Geometry: see drawing. Coordinates: mm, zero at the bounding-box minimum. A direction names the side the tool comes from. Coordinates: 2 decimals unless noted, no trailing zeros. Write each loop counter-clockwise with the first axis right and the second up, starting at its lowest first coordinate (ties: lowest second). Pieces come first, ordered by that corner, then holes. Notation, with made-up numbers: M -22,17.25 L 34,17.25 A18 ccw 34,26.25 Z; hole C 76,9.25 d2. An arc over 180 degrees is marked long. One line per item, written item: value. Start each with the question number.
Item 1: Cut plane C-C, the plane y = 45. Output: boundary loops of the cut face in (x, z).
Item 2: Cut plane A-A, the plane z = 20.32. Output: boundary loops of the cut face in (x, y).
Item 3: Set-up query: the marked faces 1 and 2. Return all of +Z, -Z, +X, -X, +Y, -Y with unobstructed straight access to the full face (end or side cutting, diameter ignored); none if empty.
Item 4: Cut plane B-B, the plane x = 0.75. Output: boundary loops of the cut face in (y, z), then the cut area to 3 significant figures.
Item 5: Mould query, pull axis Z, two halves, no side actions, for the marked faces 3, 4, 5 and 6. Classes: released by +Z, released by -Z, zero draft, split by the parting line, or undercut.
Item 6: Cut plane D-D, the plane z = 38.5. Output: boundary loops of the cut face in (x, y).
Item 7: Pin query (flat end, axial travel): P1, Ø1, axis at x = 3, z = 36, coming from the +Y side; P2, Ø1.9, axis at x = 4.5, z = 23, coming from the -Y side. Return the tip coordinate at first contact, or that it passes through.
Item 8: Ray query, L1, parallel to Y at x = 4, z = 20.32; L2, parallel to Z at x = 5.75, y = 3; L3, parallel to Y at x = 4, z = 18. Return the intervals inside material, ascending. Write a range as from..to.
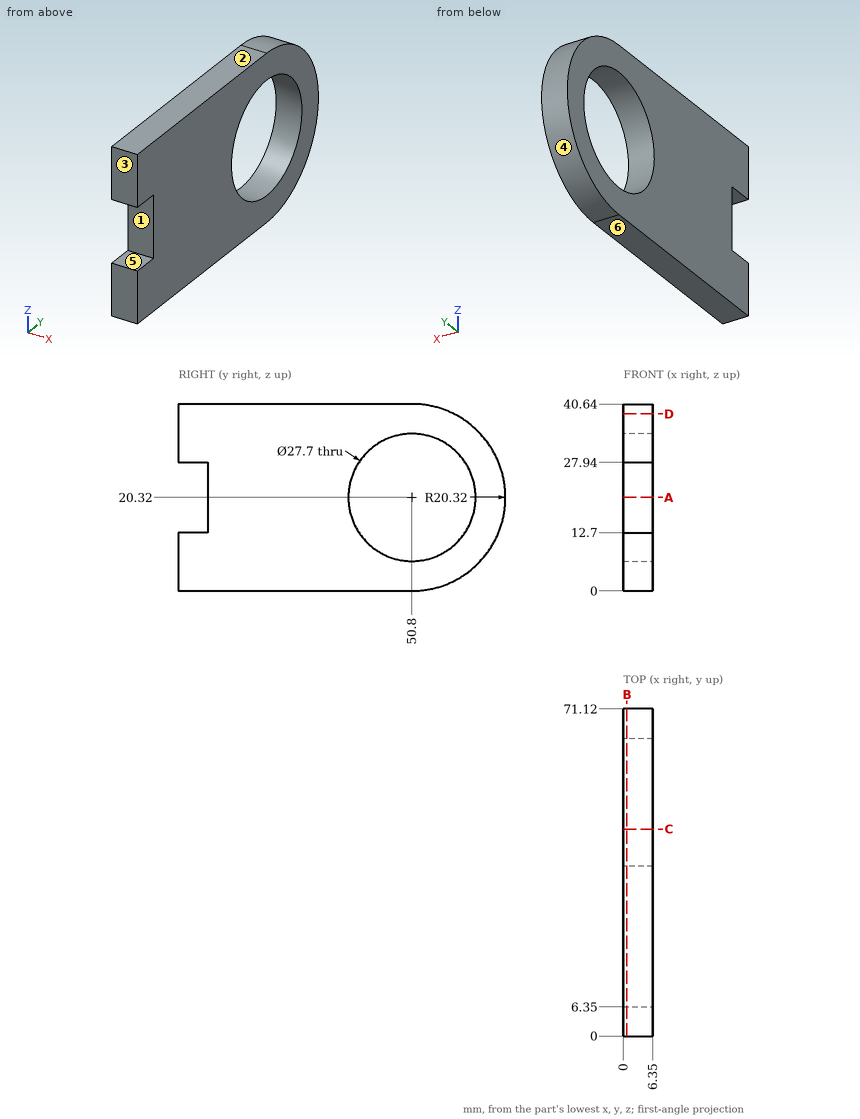
From the geometry:
1. outline: M 0,0 L 6.35,0 L 6.35,7.74 L 0,7.74 Z; M 0,32.9 L 6.35,32.9 L 6.35,40.64 L 0,40.64 Z
2. outline: M 0,6.35 L 6.35,6.35 L 6.35,36.95 L 0,36.95 Z; M 0,64.65 L 6.35,64.65 L 6.35,71.12 L 0,71.12 Z
3. face 1: +X, -X, -Y
3. face 2: +Z, +X, -X, +Y, -Y
4. outline: M 0,0 L 50.8,0 A20.32 ccw 50.8,40.64 L 0,40.64 L 0,27.94 L 6.35,27.94 L 6.35,12.7 L 0,12.7 Z; hole C 50.8,20.32 d27.7
4. area: 2,010 mm²
5. face 3: zero draft
5. face 4: split by the parting line
5. face 5: undercut
5. face 6: released by -Z
6. outline: M 0,0 L 6.35,0 L 6.35,59.88 L 0,59.88 Z
7. P1: stops at y = 64.31
7. P2: stops at y = 6.35
8. L1: y = 6.35..36.95, 64.65..71.12
8. L2: z = 0..12.7, 27.94..40.64
8. L3: y = 6.35..37.15, 64.45..70.99
